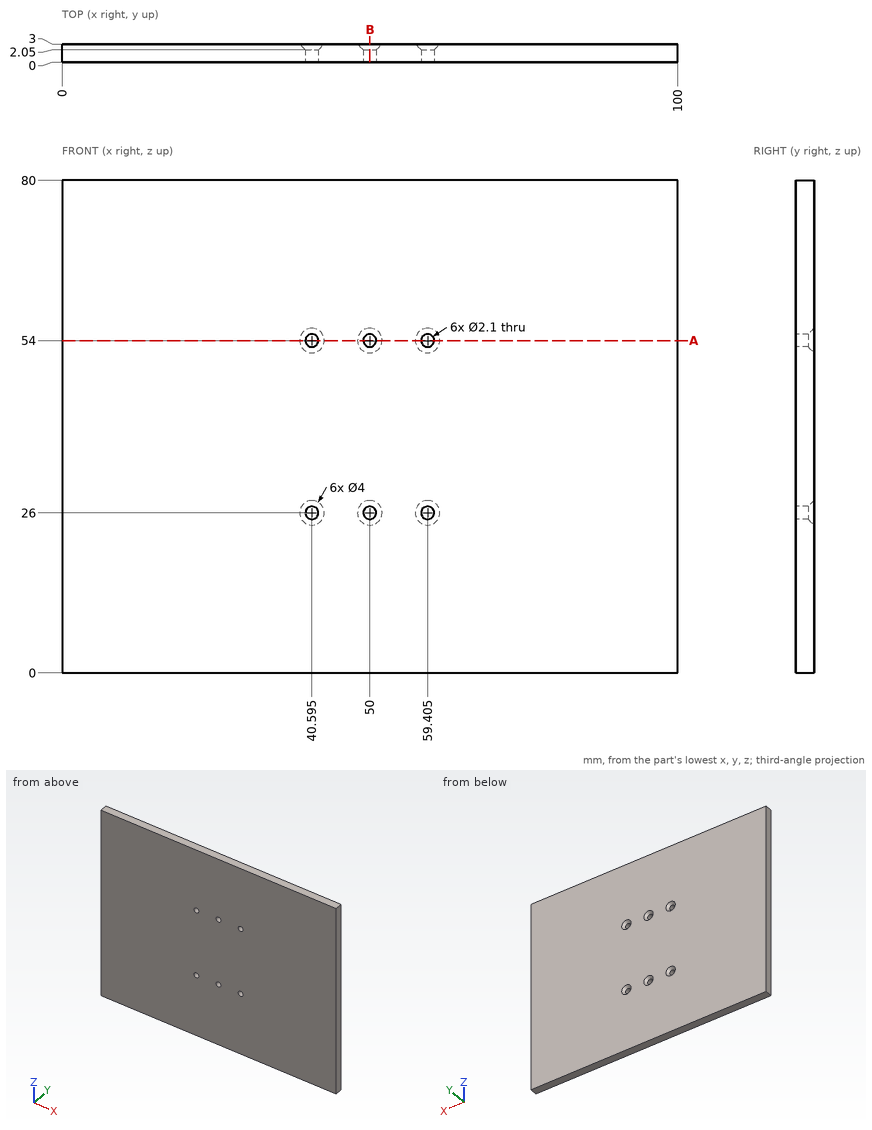
Could you check a few things on this drawing? It's one solid part, dimensions in mm from its lowest x, y, z. Coordinates: 2 decimals unless noted, no trailing zeros. Order: outer loops, then holes, each group sorted by start corner. A loop starts at its lowest first (then second) coordinate and runs counter-clockwise, first axis right, second up. Notation, with made-up numbers: (-10, 13.25) - (23, 13.25) arc R31 cw to (23, 43.25) - close; hole circle Ø2 at (11.5, 83). An arc over 180 degrees is marked (long way). One line per question, with ' | ' between items. Start each with the question number.
1. If we section it at B-B (x = 50): Write out the boundary of the cut face in (y, z), and give its area (3 significant figures).
2. If we section it at A-A (z = 54): Write out the boundary of the cut face in (x, y) (3 decimals), and give its area (3 significant figures).
3. Please list where this line runs through material, in increasing order: line 1 along X through (y, z) = (0.7, 26) (3 decimals). Write a range as [from, to].
4. I'm going to push flat-ended pins straight in: pin 1 Ø2.5 at (x, z) = (40.595, 26) entering from +Y; pin 2 Ø1.7 at (x, z) = (50, 54) entering from +Y; pin 3 Ø3.5 at (x, z) = (50, 26) entering from +Y. Where does each tip first touch, or does it pass through?
Model answer:
1) outline: (0, 0) - (3, 0) - (3, 24) - (2.05, 24.95) - (0, 24.95) - close; (0, 27.05) - (2.05, 27.05) - (3, 28) - (3, 52) - (2.05, 52.95) - (0, 52.95) - close; (0, 55.05) - (2.05, 55.05) - (3, 56) - (3, 80) - (0, 80) - close | area: 226 mm²
2) outline: (0, 0) - (39.545, 0) - (39.545, 2.05) - (38.595, 3) - (0, 3) - close; (41.645, 0) - (48.95, 0) - (48.95, 2.05) - (48, 3) - (42.595, 3) - (41.645, 2.05) - close; (51.05, 0) - (58.355, 0) - (58.355, 2.05) - (57.405, 3) - (52, 3) - (51.05, 2.05) - close; (60.455, 0) - (100, 0) - (100, 3) - (61.405, 3) - (60.455, 2.05) - close | area: 278 mm²
3) line 1: x = [0, 39.545], [41.645, 48.95], [51.05, 58.355], [60.455, 100]
4) pin 1: stops at y = 2.25 | pin 2: passes through | pin 3: stops at y = 2.75
